```python
from build123d import *

# Parameters (mm, degrees)
ESQUISSE1_W             = 38
ESQUISSE1_H             = 23
BOSS_EXTRU_1_DEPTH      = 100.3
ESQUISSE4_R             = 16.1
ENL_V_MAT_EXTRU_1_DEPTH = 101.3
ESQUISSE5_W             = 65
ESQUISSE5_H             = 6.5
ENL_V_MAT_EXTRU_2_DEPTH = 39


with BuildPart() as part:
    # Esquisse1 → Boss.-Extru.1 (new body)
    with BuildSketch(Plane.XY):
        with Locations((19, 11.5)):
            Rectangle(ESQUISSE1_W, ESQUISSE1_H)
    extrude(amount=BOSS_EXTRU_1_DEPTH)

    # Esquisse4 → Enlèv. mat.-Extru.1 (cut, through all)
    with BuildSketch(Plane.XY):
        with Locations((19, 23)):
            Circle(ESQUISSE4_R)
    extrude(amount=ENL_V_MAT_EXTRU_1_DEPTH, mode=Mode.SUBTRACT)

    # Esquisse5 → Enlèv. mat.-Extru.2 (cut, through all)
    with BuildSketch(Plane(origin=(0, 0, 0), x_dir=(0, 0, -1), z_dir=(1, 0, 0))):
        with Locations((-44.225007926, 3.25)):
            Rectangle(ESQUISSE5_W, ESQUISSE5_H)
    extrude(amount=ENL_V_MAT_EXTRU_2_DEPTH, mode=Mode.SUBTRACT)


solid = part.part
```
Model file for the job. Use its own axes, mm. A direction names the side the tool comes from. Give positions to 0.01 mm unless a question says otherwise; leave off trailing zeros. Write each loop counter-clockwise with the first axis right and the second up, starting at its lowest first coordinate (ties: lowest second). Pieces come first, ordered by that corner, then holes. Notation, with made-up numbers: (-38.5, 4.5) - (15.5, 4.5) arc R11 cw to (15.5, 25.5) - close; hole circle Ø2 at (34.25, 30). An arc over 180 degrees is marked (long way). One line per question, with ' | ' between items. Start each with the question number.
(1) Slice it at A-A on y = 19.25. Write the cut outline in (x, z), plus the area to 3 significant figures.
(2) Slice it at C-C on z = 35. Write the cut outline in (x, y), plus the area to 3 significant figures.
(3) Slice it at B-B on x = 19. Write the cut outline in (y, z) (3 decimals).
(4) Two-plate mould, pull along Z, no slides. Class faces 3 (the face through (1, 23, 49)), 4 (the face through (18.7, 6.5, 0)), 5 (the face through (19, 6.5, 45)), 6 (the face through (18.7, 6.5, 100.3)): +Z half, -Z half, draft (parallel to the pull), parting line (faces both ways), or undercut.
(5) Slice it at D-D on y = 8.25. Write the cut outline in (x, z), plus the area to 3 significant figures.
(6) Pin check, flat tips, straight feed: P1, Ø11.5, axis at x = 24, z = 58, coming from the -Y side; P2, Ø10, axis at x = 14.5, z = 88, coming from the +Y side. Stop position of each tip, or through.
(7) Wall check: line 1 along Z through (x, y) = (20.5, 3.5) (3 decimals); line 2 along X through (y, z) = (19.25, 72); line 3 along X through (y, z) = (21.5, 60). Give the ranges that are in metal, low to high. Write a range as from..to.
(8) 3-axis set-ups, long thin cutter, end or side, ignore diameter. For faces 1 (the face through (37, 23, 49)), 2 (the face through (19, 3, 11.725)): which of +Z, -Z, +X, -X, +Y, -Y reach the whole face in a straight line?
Results below:
1) outline: (0, 0) - (3.34, 0) - (3.34, 100.3) - (0, 100.3) - close; (34.66, 0) - (38, 0) - (38, 100.3) - (34.66, 100.3) - close | area: 671 mm^2
2) outline: (0, 6.5) - (38, 6.5) - (38, 23) - (35.1, 23) arc R16.1 cw to (2.9, 23) - (0, 23) - close | area: 220 mm^2
3) outline: (0, 0) - (6.9, 0) - (6.9, 100.3) - (0, 100.3) - (0, 76.725) - (6.5, 76.725) - (6.5, 11.725) - (0, 11.725) - close
4) face 3: draft | face 4: -Z half | face 5: undercut | face 6: +Z half
5) outline: (0, 0) - (12.55, 0) - (12.55, 100.3) - (0, 100.3) - close; (25.45, 0) - (38, 0) - (38, 100.3) - (25.45, 100.3) - close | area: 2,520 mm^2
6) P1: y = 6.5 | P2: y = 10
7) line 1: 0..11.725, 76.725..100.3 | line 2: 0..3.34, 34.66..38 | line 3: 0..2.97, 35.03..38
8) face 1: +Z, -Z, +X, -X, +Y | face 2: +X, -X, -Y
